```python
from build123d import *

# Parameters (mm, degrees)
EXTRUDE_START       = 10
SKETCH_1_R          = 12.5
EXTRUDE_1_DEPTH     = 150
SKETCH_2_W          = 9.934119033
SKETCH_2_H          = 36.471756902
CUT_EXTRUDE_1_DEPTH = 35


with BuildPart() as part:
    # Эскиз1 → Вытянуть1 (new body)
    with BuildSketch(Plane.XY.offset(EXTRUDE_START)):
        Circle(SKETCH_1_R)
    extrude(amount=EXTRUDE_1_DEPTH)

    # Эскиз2 → Вырез-Вытянуть1 (cut, symmetric)
    with BuildSketch(Plane(origin=(0, 0, 0), x_dir=(1, 0, 0), z_dir=(0, 1, 0))):
        with Locations((-0.001487871, -170.197950686)):
            Rectangle(SKETCH_2_W, SKETCH_2_H)
    extrude(amount=CUT_EXTRUDE_1_DEPTH, both=True, mode=Mode.SUBTRACT)


solid = part.part
```
Work out the finished part from the listing and answer in its coordinate system (mm). A direction names the side the tool comes from. Coordinates: 2 decimals unless noted, no trailing zeros. Order: outer loops, then holes, each group sorted by start corner. A loop starts at its lowest first (then second) coordinate and runs counter-clockwise, first axis right, second up. Notation, with made-up numbers: M 82,81.25 L 89,81.25 A26 cw 89,102.25 Z; hole C -24,-25.5 d1. An arc over 180 degrees is marked long. Use CSV: the item, a comma, the result in double quotes.
1) Section C-C on z = 135 is taken. Write down the section's boundary in (x, y), plus the area to 3 significant figures.
Worked out:
outline,"C 0,0 d25"
area,"491 mm^2"
2) Section A-A on y = 0 is taken. Write down the section's boundary in (x, z), plus the area to 3 significant figures.
Worked out:
outline,"M -12.5,10 L 12.5,10 L 12.5,160 L 4.97,160 L 4.97,151.96 L -4.97,151.96 L -4.97,160 L -12.5,160 Z"
area,"3,670 mm^2"
3) Section B-B on x = 0 is taken. Write down the section's boundary in (y, z), plus the area to 3 significant figures.
Worked out:
outline,"M -12.5,10 L 12.5,10 L 12.5,151.96 L -12.5,151.96 Z"
area,"3,550 mm^2"
4) Flat-ended cylindrical pins translate along their axes: pin 1 Ø3 at (x, z) = (3, 48) entering from -Y; pin 2 Ø8 at (x, z) = (5, 57) entering from -Y; pin 3 Ø2 at (y, z) = (-8.5, 124) entering from +X. Find the tip coordinate at first contact, or state that the pin passes through.
Worked out:
pin 1,"stops at y = -12.41"
pin 2,"stops at y = -12.46"
pin 3,"stops at x = 10"
5) For faces 4 (the face through (8, 0, 160)), 5 (the face through (4.966, 0, 156)), determine the directions among +Z, -Z, +X, -X, +Y, -Y from which every point of the face is accessible in a straight line to the end or side of a thin tool.
Worked out:
face 4,"+Z, +X, -X, +Y, -Y"
face 5,"+Z, +Y, -Y"
6) Determine the mould class of faces 1 (the face through (0, 0, 10)), 2 (the face through (0, 0, 151.962)), 3 (the face through (11.923, 3.755, 83.95)) for opening direction X: released by +X, released by -X, zero draft, split by the parting line, or undercut.
Worked out:
face 1,"zero draft"
face 2,"undercut"
face 3,"split by the parting line"
7) Section D-D on y = -9.75 is taken. Write down the section's boundary in (x, z).
Worked out:
outline,"M -7.82,10 L 7.82,10 L 7.82,160 L 4.97,160 L 4.97,151.96 L -4.97,151.96 L -4.97,160 L -7.82,160 Z"
8) Consider line 1 (Z direction, x = 4.25, y = 10.25); line 2 (X direction, y = -4.25, z = 50.5); line 3 (Y direction, x = 6, z = 128). Determine where each line is inside the solid, lowest interval first. Write a range as [from, to].
Worked out:
line 1,"z = [10, 151.96]"
line 2,"x = [-11.76, 11.76]"
line 3,"y = [-10.97, 10.97]"
